Geometry: final body of the model. Coordinates: model frame, mm. A direction names the side the tool comes from. Coordinates: 2 decimals unless noted, no trailing zeros. Loops run counter-clockwise (first coordinate to the right, second up) from the corner with the lowest first, then second, coordinate; pieces in that order, holes last. Notation, with made-up numbers: (-14, 8) - (18, 8) arc R15 ccw to (18, 16) - close; hole circle Ø10 at (68, 65.25). An arc over 180 degrees is marked (long way). Return JSON: item names as keys, results as strings.
from build123d import *

# Parameters (mm, degrees)
SKETCH1_R           = 3.75
BOSS_EXTRUDE1_DEPTH = 7.25
SKETCH2_R           = 3.75
SKETCH2_R_2         = 2.5
CUT_EXTRUDE1_DEPTH  = 4
SKETCH3_R           = 1.65
BOSS_EXTRUDE2_DEPTH = 2


with BuildPart() as part:
    # Sketch1 → Boss-Extrude1 (new body)
    with BuildSketch(Plane(origin=(0, 0, 0), x_dir=(1, 0, 0), z_dir=(0, 1, 0))):
        Circle(SKETCH1_R)
    extrude(amount=BOSS_EXTRUDE1_DEPTH)

    # Sketch2 → Cut-Extrude1 (cut)
    with BuildSketch(Plane(origin=(0, 7.25, 0), x_dir=(1, 0, 0), z_dir=(0, 1, 0))):
        Circle(SKETCH2_R)
        Circle(SKETCH2_R_2, mode=Mode.SUBTRACT)
    extrude(amount=-CUT_EXTRUDE1_DEPTH, mode=Mode.SUBTRACT)

    # Sketch3 → Boss-Extrude2 (add)
    with BuildSketch(Plane(origin=(0, 7.25, 0), x_dir=(1, 0, 0), z_dir=(0, 1, 0))):
        Circle(SKETCH3_R)
    extrude(amount=BOSS_EXTRUDE2_DEPTH)


solid = part.part
Item 1: Section query D-D, the plane z = -2. Return loops of the section in (x, y), and give its area (3 significant figures).
Worked out:
{"outline": "(-3.17, 0) - (3.17, 0) - (3.17, 3.25) - (1.5, 3.25) - (1.5, 7.25) - (-1.5, 7.25) - (-1.5, 3.25) - (-3.17, 3.25) - close", "area": "32.6 mm^2"}
Item 2: Section query A-A, the plane z = 0. Return loops of the section in (x, y).
Worked out:
{"outline": "(-3.75, 0) - (3.75, 0) - (3.75, 3.25) - (2.5, 3.25) - (2.5, 7.25) - (1.65, 7.25) - (1.65, 9.25) - (-1.65, 9.25) - (-1.65, 7.25) - (-2.5, 7.25) - (-2.5, 3.25) - (-3.75, 3.25) - close"}
Item 3: Ray query, probe 1 along Y at (x, z) = (2, 2.5); probe 2 along Y at (x, z) = (1.25, -1.5); probe 3 along X at (y, z) = (5.5, -2). Return the intervals inside material, ascending. Write a range as from..to.
Worked out:
{"probe 1": "0..3.25", "probe 2": "0..7.25", "probe 3": "-1.5..1.5"}
Item 4: First-contact query: pin 1 Ø3 at (x, z) = (-1.5, -2) entering from +Y; pin 2 Ø4 at (x, y) = (-0.5, 7) entering from +Z; pin 3 Ø1 at (x, y) = (1.5, 3) entering from -Z. Flat tips, straight axial feed; report the tip coordinate or a pass-through.
Worked out:
{"pin 1": "y = 9.25", "pin 2": "z = 2.5", "pin 3": "z = -3.61"}
Item 5: Section query B-B, the plane x = 0. Return loops of the section in (y, z).
Worked out:
{"outline": "(0, -3.75) - (3.25, -3.75) - (3.25, -2.5) - (7.25, -2.5) - (7.25, -1.65) - (9.25, -1.65) - (9.25, 1.65) - (7.25, 1.65) - (7.25, 2.5) - (3.25, 2.5) - (3.25, 3.75) - (0, 3.75) - close"}
Item 6: Reachability of faces 1 (the face through (-3.746, 1.602, -0.165)), 2 (the face through (-1.216, 8.236, -1.115)) from +Z, -Z, +X, -X, +Y, -Y: full face, straight path, thin tool, end or side. Return the list, or none.
Worked out:
{"face 1": "+Y, -Y", "face 2": "+Y"}
Item 7: Section query C-C, the plane y = 2. Return loops of the section in (x, z), and give its area (3 significant figures).
Worked out:
{"outline": "circle Ø7.5 at (0, 0)", "area": "44.2 mm^2"}
